from build123d import *

# Parameters (mm, degrees)
SKETCH1_R           = 10
BOSS_EXTRUDE1_DEPTH = 550
SKETCH4_R           = 7.5
BOSS_EXTRUDE2_DEPTH = 40
SKETCH5_R           = 6
BOSS_EXTRUDE3_DEPTH = 12
CHAMFER1_SIZE       = 0.5


with BuildPart() as part:
    # Sketch1 → Boss-Extrude1 (new body)
    with BuildSketch(Plane.XY):
        Circle(SKETCH1_R)
    extrude(amount=BOSS_EXTRUDE1_DEPTH)

    # Sketch4 → Boss-Extrude2 (add)
    with BuildSketch(Plane.XY.offset(550)):
        Circle(SKETCH4_R)
    extrude(amount=BOSS_EXTRUDE2_DEPTH)

    # Sketch5 → Boss-Extrude3 (add)
    with BuildSketch(Plane.XY.offset(590)):
        Circle(SKETCH5_R)
    extrude(amount=BOSS_EXTRUDE3_DEPTH)

    # Chamfer1
    chamfer1_edges = [part.edges().sort_by_distance(p)[0] for p in [
        (-6, 0, 602),
        (-10, 0, 0),
        (-10, 0, 550),
        (-7.5, 0, 590),
    ]]
    chamfer(chamfer1_edges, length=CHAMFER1_SIZE)


solid = part.part
Read the model definition and answer for the solid it produces. Units are mm, in the model's axes. A direction names the side the tool comes from. Round coordinates to 2 decimals unless told otherwise and drop trailing zeros. Write each loop counter-clockwise with the first axis right and the second up, starting at its lowest first coordinate (ties: lowest second). Pieces come first, ordered by that corner, then holes.
1. The part is cut by section C-C, the plane z = 117.5. Determine the outline of the cut face in (x, y), then the cut area to 3 significant figures.
2. Which of the six approach directions +Z, -Z, +X, -X, +Y, -Y give full straight-line access (tool end or side, diameter ignored) to faces 4 (the face through (0, 0, 602)), 5 (the face through (6, 2, 590))?
3. Straight lines are drawn through the part: L1, parallel to X at y = -1, z = 139.5; L2, parallel to Z at x = -2, y = -6.75. For each, find the intervals that lie inside material, in ascending order.
4. Given pin 1 Ø5 at (x, z) = (7.5, 135.5) entering from +Y; pin 2 Ø8 at (x, z) = (7.5, 242.5) entering from +Y; pin 3 Ø1 at (y, z) = (6, 318) entering from -X, each flat-ended and moving along its own axis, determine where each tip first touches the part or whether it passes through.
5. The part is cut by section A-A, the plane y = 0. Determine the outline of the cut face in (x, z).
6. Determine the mould class of faces 1 (the face through (0, 0, 0)), 2 (the face through (1, 8, 550)), 3 (the face through (-6, 0, 596)) for opening direction Z: pulls with the +Z half, pulls with the -Z half, needs draft (parallel to the pull), parting line crosses it, or undercut.
Values:
1. outline: circle Ø20 at (0, 0)
1. area: 314 mm2
2. face 4: +Z, +X, -X, +Y, -Y
2. face 5: +Z
3. L1: x = -9.95 to 9.95
3. L2: z = 0 to 589.96
4. pin 1: stops at y = 8.66
4. pin 2: stops at y = 9.37
4. pin 3: stops at x = -8.35
5. outline: (-10, 0.5) - (-9.5, 0) - (9.5, 0) - (10, 0.5) - (10, 549.5) - (9.5, 550) - (7.5, 550) - (7.5, 589.5) - (7, 590) - (6, 590) - (6, 601.5) - (5.5, 602) - (-5.5, 602) - (-6, 601.5) - (-6, 590) - (-7, 590) - (-7.5, 589.5) - (-7.5, 550) - (-9.5, 550) - (-10, 549.5) - close
6. face 1: pulls with the -Z half
6. face 2: pulls with the +Z half
6. face 3: needs draft
